Autodesk Inventor part; units mm, degrees
ref_plane "YZ Plane" through (0, 0, 0) normal (1, 0, 0) x (0, 1, 0)
ref_plane "XZ Plane" through (0, 0, 0) normal (0, 1, 0) x (-1, 0, 0)
ref_plane "XY Plane" through (0, 0, 0) normal (0, 0, 1) x (1, 0, 0)
sketch "Sketch1" plane through (0, 0, 0) normal (0, 1, 0) x (-1, 0, 0)
  line L0 (0, 0) -> (127, 0)
  line L1 (127, 0) -> (127, -127)
  line L2 (127, -127) -> (0, -127)
  line L3 (0, -127) -> (0, 0)
  dimension "d0" = 127
  dimension "d1" = 127
extrude "Extrusion1" add sketch "Sketch1" along normal blind 254
sketch "Sketch3" plane through (0, 0, 0) normal (0, -1, 0) x (1, 0, 0)
  line L0 (0, -127) -> (-127, -127)
  line L1 (-127, -127) -> (-127, 0)
  line L2 (0, 0) -> (0, -127)
  line L3 (-127, 0) -> (0, 0)
  circle A0 centre (-31.75, -31.75) radius 6.35
  circle A1 centre (-95.25, -31.75) radius 6.35
  circle A2 centre (-95.25, -95.25) radius 6.35
  circle A3 centre (-31.75, -95.25) radius 6.35
  dimension "d5" = 12.7
  dimension "d6" = 12.7
  dimension "d7" = 12.7
  dimension "d8" = 12.7
extrude "Extrusion2" add sketch "Sketch3" along normal blind 25.4 contours A0 | A1 | A2 | A3
thread "Thread1"
thread "Thread2"
thread "Thread3"
thread "Thread4"
chamfer "Chamfer1" distance 25.4 angle 45 1 edges at (-63.5, 254, -127)
sketch "Sketch5" plane through (0, 0, 0) normal (1, 0, 0) x (0, 0, -1)
  line L0 (127, 0) -> (127, 228.6)
  line L1 (101.6, 254) -> (0, 254)
  line L2 (12.7, 223.2608) -> (88.9, 223.2608)
  line L3 (88.9, 223.2608) -> (88.9, 248.6608)
  line L4 (88.9, 248.6608) -> (12.7, 248.6608)
  line L5 (12.7, 248.6608) -> (12.7, 223.2608)
  line L6 (12.7, 223.2608) -> (88.9, 248.6608) construction
  line L7 (88.9, 223.2608) -> (12.7, 248.6608) construction
  point P0 (0, 0)
  point P1 (50.8, 235.9608)
  dimension "d22" = 76.2
  dimension "d23" = 25.4
extrude "Extrusion3" add sketch "Sketch5" along normal blind 254
sketch "Sketch6" plane through (0, 248.6608, -12.7) normal (0, 1, 0) x (1, 0, 0)
  line L0 (0, 0) -> (254, 0)
  line L1 (254, 0) -> (203.2, 0)
  line L2 (203.2, 0) -> (203.2, 76.2)
  line L3 (203.2, 76.2) -> (254, 76.2)
  line L4 (254, 76.2) -> (254, 0)
  point P0 (0, -12.7)
  dimension "d26" = 50.8
  dimension "d27" = 76.2
extrude "Extrusion4" add sketch "Sketch6" along normal blind 152.4
sketch "Sketch7" plane through (203.2, 248.6608, -88.9) normal (-1, 0, 0) x (0, 0, 1)
  line L0 (0, 152.4) -> (76.2, 152.4)
  line L1 (38.1, 152.4) -> (38.1, 120.65)
  circle A0 centre (38.1, 120.65) radius 25.4
  point P0 (88.9, -248.6608)
  dimension "d30" = 31.75
  dimension "d31" = 50.8
extrude "Extrusion5" cut sketch "Sketch7" against normal blind 38.1
sketch "Sketch8" plane through (-127, 0, -127) normal (-1, 0, 0) x (0, 0, 1)
  line L0 (114.3, 223.2608) -> (114.3, 248.6608)
  line L1 (114.3, 248.6608) -> (38.1, 248.6608)
  line L2 (38.1, 223.2608) -> (114.3, 223.2608)
  line L3 (114.3, 223.2608) -> (114.3, 248.6608)
  line L4 (114.3, 248.6608) -> (38.1, 248.6608)
  line L5 (38.1, 248.6608) -> (38.1, 223.2608)
  line L6 (38.1, 223.2608) -> (114.3, 223.2608)
  line L7 (25.4, 254) -> (0, 228.6)
  line L8 (127, 254) -> (25.4, 254)
  line L9 (127, 0) -> (127, 254)
  line L10 (0, 0) -> (127, 0)
  line L11 (0, 0) -> (0, 228.6)
extrude "Extrusion6" add sketch "Sketch8" along normal blind 254 contours L2 L5 L1 L0
sketch "Sketch9" plane through (-127, 248.6608, -12.7) normal (0, 1, 0) x (1, 0, 0)
  line L0 (0, 76.2) -> (0, 0)
  line L1 (0, 76.2) -> (-254, 76.2)
  line L2 (-254, 0) -> (-254, 76.2)
  line L3 (0, 0) -> (-254, 0)
  line L4 (-254, 76.2) -> (-254, 0)
  line L5 (-254, 0) -> (-203.2, 0)
  line L6 (-203.2, 0) -> (-203.2, 76.2)
  line L7 (-203.2, 76.2) -> (-254, 76.2)
  line L8 (-254, 76.2) -> (-254, 0)
  point P0 (127, -12.7)
  dimension "d36" = 50.8
  dimension "d37" = 76.2
extrude "Extrusion7" add sketch "Sketch9" along normal blind 152.4 contours L6 L3 L2 L1
sketch "Sketch10" plane through (-330.2, 248.6608, -12.7) normal (1, 0, 0) x (0, 0, -1)
  circle A0 centre (38.1, 120.65) radius 25.4
  circle A1 centre (38.1, 120.65) radius 25.4
  point P0 (-12.7, -248.6608)
extrude "Extrusion8" cut sketch "Sketch10" against normal blind 38.1
properties part number "TubePostV1"
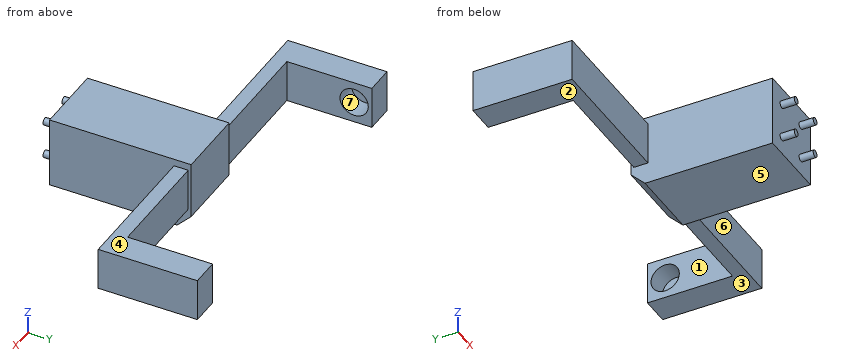
Geometry check sheet. Reference: the model listing, model coordinates, mm. Face numbers are marked on the shaded views. A direction names the side the tool comes from. Give positions to 0.01 mm unless a question says otherwise; leave off trailing zeros. Order: outer loops, then holes, each group sorted by start corner. A loop starts at its lowest first (then second) coordinate and runs counter-clockwise, first axis right, second up. Notation, with made-up numbers: (8, 30) - (21, 30) arc R22 ccw to (21, 69) - close; hole circle Ø4 at (-8, 35). An arc over 180 degrees is marked (long way). Answer in a Markdown table with one row per item. Add a question column.
Q1. Material ranges on probe 1 along Y at (x, z) = (-348, -50); probe 2 along X at (y, z) = (374, -35); probe 3 along X at (y, z) = (321.5, -28), recorded low to high. Write a range as from..to.
Q2. Cross-section at C-C, the plane y = 21. Enter the section's corners in (x, z).
Q3. Mould release check, pull along Z, two halves, no side actions. Record for the marked faces 5, 6 and 7: pulls with the +Z half, pulls with the -Z half, needs draft (parallel to the pull), parting line crosses it, or undercut.
Q4. Cross-section at B-B, the plane z = -50.8. Enter the section's corners in (x, y).
Q5. Tool access check on the marked faces 1, 2, 3 and 4. Record the directions out of +Z, -Z, +X, -X, +Y, -Y that give a thin tool (end or side, any length) a straight path to the whole face; none if there is none.
Q6. Cross-section at A-A, the plane x = -31.75. Enter the section's corners in (y, z).
Q7. Gauge pin test, flat ends, axial feed: pin 1 (23 mm diameter, centred on x = -233.5, z = -54, fed in from +Y); pin 2 (1 mm diameter, centred on y = 38, z = -92.5, fed in from -X); pin 3 (12 mm diameter, centred on x = 159, z = -18, fed in from -Y). Record the tip position at first contact, or that the pin passes through.
Q8. Cross-section at D-D, the plane x = -339.5. Enter the section's corners in (y, z).
Check values:
| question | item | result |
|---|---|---|
| 1 | probe 1 | y = 223.26..343.92, 394.7..401.06 |
| 1 | probe 2 | x = -381..-368.3, 241.3..254 |
| 1 | probe 3 | x = -381..-330.2, 203.2..254 |
| 2 | outline | (-127, -127) - (0, -127) - (0, 0) - (-127, 0) - close |
| 3 | face 5 | pulls with the -Z half |
| 3 | face 6 | needs draft |
| 3 | face 7 | undercut |
| 4 | outline | (-381, 223.26) - (-127, 223.26) - (-127, 0) - (0, 0) - (0, 223.26) - (254, 223.26) - (254, 401.06) - (203.2, 401.06) - (203.2, 394.71) - (241.3, 394.71) - (241.3, 343.91) - (203.2, 343.91) - (203.2, 248.66) - (0, 248.66) - (0, 254) - (-127, 254) - (-127, 248.66) - (-330.2, 248.66) - (-330.2, 343.91) - (-368.3, 343.91) - (-368.3, 394.71) - (-330.2, 394.71) - (-330.2, 401.06) - (-381, 401.06) - close |
| 5 | face 1 | +Z, -Z, +Y |
| 5 | face 2 | -Z, -X, +Y, -Y |
| 5 | face 3 | -Z, +X, +Y, -Y |
| 5 | face 4 | +Z, +X, +Y, -Y |
| 6 | outline | (-25.4, -101.6) - (0, -101.6) - (0, -127) - (228.6, -127) - (254, -101.6) - (254, 0) - (0, 0) - (0, -25.4) - (-25.4, -25.4) - (-25.4, -38.1) - (0, -38.1) - (0, -88.9) - (-25.4, -88.9) - close |
| 7 | pin 1 | stops at y = 248.66 |
| 7 | pin 2 | stops at x = -127 |
| 7 | pin 3 | stops at y = 223.26 |
| 8 | outline | (223.26, -88.9) - (401.06, -88.9) - (401.06, -12.7) - (223.26, -12.7) - close; hole circle Ø50.8 at (369.31, -50.8) |
